Autodesk Inventor part; units mm, degrees
ref_plane "YZ Plane" through (0, 0, 0) normal (1, 0, 0) x (0, 1, 0)
ref_plane "XZ Plane" through (0, 0, 0) normal (0, 1, 0) x (-1, 0, 0)
ref_plane "XY Plane" through (0, 0, 0) normal (0, 0, 1) x (1, 0, 0)
sketch "Sketch1" plane through (0, 0, 0) normal (0, 1, 0) x (-1, 0, 0)
  line L0 (55, 27.5) -> (-55, 27.5)
  line L1 (-55, 27.5) -> (-55, -27.5)
  line L2 (-55, -27.5) -> (55, -27.5)
  line L3 (55, -27.5) -> (55, 27.5)
  point P0 (0, 0)
  point P1 (-55, 0)
  point P2 (55, 0)
  dimension "d0" = 55
  dimension "d66" = 27.5
  dimension "d67" = 55
  dimension "d68" = 55
extrude "Extrusion1" add sketch "Sketch1" along normal blind 21
sketch "Sketch2" plane through (0, 21, 0) normal (0, 1, 0) x (1, 0, 0)
  line L0 (-55, -27.5) -> (55, -27.5)
  line L1 (55, 27.5) -> (-55, 27.5)
  line L2 (52, -27.5) -> (-50.25, -27.5)
  line L3 (-50.25, -27.5) -> (-50.25, 27.5)
  line L4 (-50.25, 27.5) -> (52, 27.5)
  line L5 (52, 27.5) -> (52, -27.5)
  line L6 (-55, 27.5) -> (-55, -27.5)
  line L7 (55, -27.5) -> (55, 27.5)
  line L8 (-50.25, 27.5) -> (52, 27.5)
  line L9 (52, 27.5) -> (52, 22.5)
  line L10 (52, 22.5) -> (-50.25, 22.5)
  line L11 (-50.25, 22.5) -> (-50.25, 27.5)
  point P0 (0, 0)
  point P1 (52, 27.5)
  point P2 (-50.25, -27.5)
  point P3 (-50.25, 22.5)
  dimension "d122" = 50.25
  dimension "d333" = 5
  dimension "d338" = 52
  dimension "d354" = 102.25
extrude "Extrusion2" cut sketch "Sketch2" against normal blind 18 contours L3 L10 L5 L0
sketch "Sketch11" plane through (0, 3, 0) normal (0, 1, 0) x (1, 0, 0)
  circle A0 centre (-12, 19) radius 1.55
  circle A1 centre (-12, -24) radius 1.55
  circle A2 centre (-46.5, 19) radius 1.55
  line L0 (-50.25, -27.5) -> (-50.25, 22.5)
  circle A3 centre (-46.5, -24) radius 1.55
  line L1 (52, -27.5) -> (-50.25, -27.5)
  line L2 (-50.25, 22.5) -> (52, 22.5)
  line L3 (-43.35, 22.5) -> (-50.25, 22.5)
  line L4 (-50.25, 22.5) -> (-50.25, 15.5)
  line L5 (-50.25, 15.5) -> (-43.35, 15.5)
  line L6 (-43.35, 15.5) -> (-43.35, 22.5)
  line L7 (-50.25, -20.5) -> (-43.35, -20.5)
  line L8 (-43.35, -20.5) -> (-43.35, -27.5)
  line L9 (-43.35, -27.5) -> (-50.25, -27.5)
  line L10 (-50.25, -27.5) -> (-50.25, -20.5)
  line L11 (-8.25, -27.5) -> (-15.15, -27.5)
  line L12 (-15.15, -27.5) -> (-15.15, -20.5)
  line L13 (-15.15, -20.5) -> (-8.25, -20.5)
  line L14 (-8.25, -20.5) -> (-8.25, -27.5)
  line L15 (-8.25, 22.5) -> (-15.15, 22.5)
  line L16 (-15.15, 22.5) -> (-15.15, 15.5)
  line L17 (-15.15, 15.5) -> (-8.25, 15.5)
  line L18 (-8.25, 15.5) -> (-8.25, 22.5)
  point P0 (-15.15, 22.5)
  dimension "d340" = 34.5
  dimension "d419" = 3.1
  dimension "d423" = 3.75
  dimension "d424" = 43
  dimension "d425" = 3.5
  dimension "d430" = 6.9
  dimension "d431" = 7
  dimension "d432" = 3.75
extrude "Extrusion17" add sketch "Sketch11" along normal blind 14
sketch "Sketch20" plane through (0, 3, 0) normal (0, 1, 0) x (1, 0, 0)
  line L0 (-50.25, -20.5) -> (-50.25, 22.5)
  line L1 (-8.25, -27.5) -> (-8.25, -20.5)
  line L2 (-8.25, -22.5) -> (52, -22.5)
  line L3 (52, -27.5) -> (-8.25, -27.5)
  line L4 (52, 22.5) -> (52, -27.5)
  point P0 (0, 0)
  point P1 (-50.25, -22.5)
  dimension "d439" = 5
extrude "Extrusion25" add sketch "Sketch20" along normal up to surface (18 mm away)
sketch "Sketch21" plane through (0, 3, 0) normal (0, 1, 0) x (1, 0, 0)
  line L0 (-43.35, -22.5) -> (-15.15, -22.5)
  line L1 (-15.15, -27.5) -> (-43.35, -27.5)
  line L2 (-43.35, -27.5) -> (-43.35, -20.5)
  line L3 (-15.15, -20.5) -> (-15.15, -27.5)
  point P0 (0, 0)
  dimension "d440" = 5
extrude "Extrusion19" add sketch "Sketch21" along normal blind 10
fillet "Fillet7" radius 2 12 edges at (-8.25, 10, -15.5) (-15.15, 10, -15.5) (-15.15, 10, 20.5) (-8.25, 10, 20.5) (-43.35, 10, 20.5) (-43.35, 10, -15.5) (-43.35, 10, -22.5) (-50.25, 10, -15.5) (-15.15, 10, -22.5) (-50.25, 10, 20.5) (-8.25, 10, -22.5) (-8.25, 10, 22.5)
sketch "Sketch23" plane through (0, 3, 0) normal (0, 1, 0) x (1, 0, 0)
  line L0 (1.75, 17) -> (42, 17)
  line L1 (42, 17) -> (42, 14)
  line L2 (42, 14) -> (1.75, 14)
  line L3 (1.75, 14) -> (1.75, 17)
  line L4 (42, -14) -> (1.75, -14)
  line L5 (1.75, -14) -> (1.75, -17)
  line L6 (1.75, -17) -> (42, -17)
  line L7 (42, -17) -> (42, -14)
  line L8 (-50.25, -27.5) -> (-50.25, 22.5)
  line L9 (-50.25, 22.5) -> (52, 22.5)
  line L10 (52, 22.5) -> (52, -22.5)
  line L11 (-8.25, 17.5) -> (-8.25, 20.5)
  line L12 (0, 0) -> (40.25, 0)
  point P0 (21.875, -14)
  point P1 (21.875, 14)
  point P2 (-52, -22.5)
  point P3 (1.75, 15.5)
  point P4 (42, 15.5)
  point P5 (21.875, -17)
  point P6 (50.25, -27.5)
  point P7 (-10.3, 15.5)
  point P8 (-8.55, 22.5)
  dimension "d375" = 3
  dimension "d380" = 3
  dimension "d433" = 10
  dimension "d434" = 10
  dimension "d438" = 28
extrude "Extrusion21" add sketch "Sketch23" along normal blind 5
fillet "Fillet8" radius 2 4 edges at (1.75, 5.5, -14) (42, 5.5, -14) (42, 5.5, 14) (1.75, 5.5, 14)
chamfer "Chamfer33" distance 2 angle 45 2 edges at (21.875, 3, 17) (21.875, 3, -17)
sketch "Sketch25" plane through (55, 0, -27.5) normal (0, 0, -1) x (-1, 0, 0)
  line L0 (76, 18.33) -> (89, 18.33)
  line L1 (89, 18.33) -> (89, 12.33)
  line L2 (89, 12.33) -> (76, 12.33)
  line L3 (76, 12.33) -> (76, 18.33)
  line L4 (110, 0) -> (110, 21)
  line L5 (0, 21) -> (110, 21)
  dimension "d411" = 6
  dimension "d412" = 13
  dimension "d447" = 21
  dimension "d448" = 2.67
extrude "Extrusion23" cut sketch "Sketch25" against normal up to surface (5 mm away)
sketch "Sketch24" plane through (-55, 0, 27.5) normal (0, 0, 1) x (1, 0, 0)
  circle A0 centre (105.6, 13) radius 2.65
  circle A1 centre (4.4, 13) radius 2.65
  circle A2 centre (105.6, 4) radius 2.65
  circle A3 centre (4.4, 4) radius 2.65
  line L0 (2.6689, 15.0064) -> (4.4, 16.5)
  line L1 (4.4, 16.5) -> (6.1311, 15.0064)
  line L2 (2.6689, 6.0064) -> (4.4, 7.5)
  line L3 (4.4, 7.5) -> (6.1311, 6.0064)
  line L4 (103.8689, 6.0064) -> (105.6, 7.5)
  line L5 (105.6, 7.5) -> (107.3311, 6.0064)
  line L6 (103.8689, 15.0064) -> (105.6, 16.5)
  line L7 (105.6, 16.5) -> (107.3311, 15.0064)
  line L8 (0, 0) -> (110, 0)
  line L9 (0, 0) -> (0, 21)
  line L10 (110, 0) -> (110, 21)
  circle A4 centre (19.05, 10.35) radius 2.65
  circle A5 centre (25.95, 10.35) radius 2.65
  circle A6 centre (32.85, 10.35) radius 2.65
  line L11 (11.65, 13) -> (39.85, 13)
  line L12 (16.4, 10.35) -> (16.4, 13)
  line L13 (21.7, 10.35) -> (21.7, 13)
  line L14 (23.3, 10.35) -> (23.3, 13)
  line L15 (28.6, 10.35) -> (28.6, 13)
  line L16 (30.2, 10.35) -> (30.2, 13)
  line L17 (35.5, 10.35) -> (35.5, 13)
  line L18 (4.75, 17) -> (11.65, 17)
  point P0 (55, 0)
  point P1 (20.0625, -1.6972)
  point P2 (19.05, 13)
  dimension "d391" = 5.3
  dimension "d399" = 3.5
  dimension "d409" = 4.4
  dimension "d410" = 4.4
  dimension "d450" = 6.9
  dimension "d451" = 6.9
  dimension "d452" = 2.65
  dimension "d453" = 4
  dimension "d454" = 19.05
  dimension "d455" = 9
extrude "Extrusion22" cut sketch "Sketch24" against normal blind 1.55
sketch "Sketch28" plane through (0, 3, 0) normal (0, 1, 0) x (1, 0, 0)
  circle A0 centre (-46.5, 19) radius 1.55
  circle A1 centre (-12, 19) radius 1.55
  circle A2 centre (-12, -24) radius 1.55
  circle A3 centre (-46.5, -24) radius 1.55
  circle A4 centre (-46.5, -24) radius 1.55
  circle A5 centre (-12, -24) radius 1.55
  circle A6 centre (-12, 19) radius 1.55
  circle A7 centre (-46.5, 19) radius 1.55
  point P0 (0, 0)
extrude "Extrusion26" add sketch "Sketch28" along normal blind 2
properties part number "PowerModuleHousing"
For this review, take the finished solid that the model builds, in its own axes (mm). A direction names the side the tool comes from. Round coordinates to 2 decimals unless told otherwise and drop trailing zeros. Order: outer loops, then holes, each group sorted by start corner. A loop starts at its lowest first (then second) coordinate and runs counter-clockwise, first axis right, second up. Notation, with made-up numbers: M -36.75,3 L -29.75,3 A7 cw -29.75,14 Z; hole C -29.5,65 d4. An arc over 180 degrees is marked long. Use a Markdown table: item, result. Add a question column.
Item 1: Add section D-D, the plane x = 0.5. Give the boundary of the cut face in (y, z), then the cut area to 3 significant figures.
Item 2: Add section B-B, the plane z = -6.5. Give the boundary of the cut face in (x, y), then the cut area to 4 significant figures.
Item 3: Insertion check: pin 1 (1 mm diameter, centred on x = -39, z = 9.5, fed in from +Y); pin 2 (2 mm diameter, centred on x = -40, y = 17, fed in from +Z); pin 3 (4 mm diameter, centred on x = 50, y = 13, fed in from +Z). Each pin has a flat end and moves straight along its axis. Give the tip position at first contact, or say it passes through.
Item 4: Add section C-C, the plane y = 4. State how many separate pieces and enclosed holes the cut face has, then the cut area to 3 significant figures.
Item 5: Add section A-A, the plane x = -22.15. Give the boundary of the cut face in (y, z).
Item 6: Mouldability with a two-part tool opening along Z and no side actions: class faces 4 (the flat face through (-34, 15, -25)), 5 (the flat face through (-15.15, 10, -19)) as released by +Z, released by -Z, zero draft, split by the parting line, or undercut.
Item 7: To check wall thickness, follow line 1 along Y through (x, z) = (50.6, 26.95); line 2 along X through (y, z) = (4, 26.8); line 3 along Z through (x, y) = (14, 6.75). State the ranges of each line that lie inside material, in increasing order.
Item 8: Tool access review of faces 1 (the cylindrical face through (-29.1, 7.7, 26.7)), 2 (the cylindrical face through (-50.69, 1.35, 26.74)), 3 (the cylindrical face through (-49.68, 10.1, 19.9)): name each direction out of +Z, -Z, +X, -X, +Y, -Y from which nothing blocks a thin tool from reaching the whole face with its end or side.
Geometry results:
| question | item | result |
|---|---|---|
| 1 | outline | M 0,-27.5 L 21,-27.5 L 21,-22.5 L 3,-22.5 L 3,22.5 L 21,22.5 L 21,27.5 L 0,27.5 Z |
| 1 | area | 345 mm² |
| 2 | outline | M -55,0 L 55,0 L 55,21 L 52,21 L 52,3 L -50.25,3 L -50.25,21 L -55,21 Z |
| 2 | area | 469.5 mm² |
| 3 | pin 1 | stops at y = 3 |
| 3 | pin 2 | stops at z = -22.5 |
| 3 | pin 3 | stops at z = 25.95 |
| 4 | separate pieces | 3 |
| 4 | enclosed holes | 1 |
| 4 | area | 1,880 mm² |
| 5 | outline | M 0,-27.5 L 12.33,-27.5 L 12.33,-22.5 L 3,-22.5 L 3,22.5 L 13,22.5 L 13,25.95 L 7.7,25.95 L 7.7,27.5 L 0,27.5 Z; M 18.33,-27.5 L 21,-27.5 L 21,-22.5 L 18.33,-22.5 Z |
| 6 | face 4 | zero draft |
| 6 | face 5 | undercut |
| 7 | line 1 | y = 0 to 1.35, 7.5 to 10.35, 16.5 to 21 |
| 7 | line 2 | x = -55 to -53.25, -47.95 to 47.95, 53.25 to 55 |
| 7 | line 3 | z = -27.5 to -22.5, -17 to -14, 14 to 17, 22.5 to 27.5 |
| 8 | face 1 | +Z, +Y |
| 8 | face 2 | +Z |
| 8 | face 3 | +Y |
